Model file for the job. Use its own axes, mm. Face numbers are marked on the shaded views. A direction names the side the tool comes from. Give positions to 0.01 mm unless a question says otherwise; leave off trailing zeros. Order: outer loops, then holes, each group sorted by start corner. A loop starts at its lowest first (then second) coordinate and runs counter-clockwise, first axis right, second up. Notation, with made-up numbers: (78.5, 36) - (116.5, 36) arc R7 ccw to (116.5, 41) - close; hole circle Ø3 at (11.25, 52). An arc over 180 degrees is marked (long way). Use CSV: the item, a comma, the result in double quotes. Start each with the question number.
(1) Band-saw the part on A-A, the plane z = 8. Give the cut face in (x, y).
(2) Band-saw the part on C-C, the plane y = -35. Give the cut face in (x, z).
(3) Pull direction Z, two halves, no side cores. Call the marked faces 5, 6 and 7: +Z half, -Z half, draft (parallel to the pull), parting line (faces both ways), or undercut.
(4) Drop flat-ended pins along their axis: pin 1 Ø3 at (x, y) = (-18, -20) entering from +Z; pin 2 Ø1.2 at (x, y) = (18, -18) entering from -Z; pin 3 Ø7.5 at (y, z) = (-5, 19.5) entering from -X; pin 4 Ø0.9 at (y, z) = (-8.5, -12) entering from +X. Give the stop position or say it passes through.
(5) Tool access for the marked faces 1, 2, 3 and 4: list every direction of +Z, -Z, +X, -X, +Y, -Y with a clear straight run to the whole face (end or side of a thin tool).
(6) Probe L1, parallel to Z at x = 18.35, y = -35; L2, parallel to X at y = -10, z = -5; L3, parallel to Z at x = 4.5, y = -11. List the from-to ranges inside material, lowest first.
(7) Band-saw the part on D-D, the plane x = 11. Give the cut face in (y, z), then the cut area to 3 significant figures.
(8) Band-saw the part on B-B, the plane y = -10.5. Give the cut face in (x, z), then the cut area to 3 significant figures.
from build123d import *

# Parameters (mm, degrees)
SKETCH_1_W                       = 35
SKETCH_1_H                       = 22
SM_BASE_FLANGE_1_DEPTH           = 1
SM_EDGE_FLANGE_1_STRIP_W         = 5
SM_EDGE_FLANGE_1_STRIP_H         = 1
SM_EDGE_FLANGE_1_STRIP_CUT_DEPTH = 22
SM_EDGE_FLANGE_1_DEPTH           = 22
SM_EDGE_FLANGE_2_STRIP_W         = 5
SM_EDGE_FLANGE_2_STRIP_H         = 1
SM_EDGE_FLANGE_2_STRIP_CUT_DEPTH = 22
SM_EDGE_FLANGE_2_DEPTH           = 22
SM_EDGE_FLANGE_3_DEPTH           = 34
EXTRUDE_1_DEPTH                  = 22
SM_EDGE_FLANGE_4_DEPTH           = 20
SM_EDGE_FLANGE_5_STRIP_CUT_DEPTH = 22
SM_EDGE_FLANGE_5_DEPTH           = 22
CUT_EXTRUDE_1_DEPTH              = 22
SKETCH_27_R                      = 1.05
CUT_EXTRUDE_2_DEPTH              = 22


# Sheet-metal steps are written as plain solids
with BuildPart() as part:
    # Sketch 1 → 基体-法兰1 (new body)
    with BuildSketch(Plane(origin=(0, 0, 0), x_dir=(1, 0, 0), z_dir=(0, 1, 0))):
        Rectangle(SKETCH_1_W, SKETCH_1_H)
    extrude(amount=-SM_BASE_FLANGE_1_DEPTH)

    # 边线-法兰1 strip (across the edge) → 边线-法兰1 strip cut (cut)
    with BuildSketch(Plane(origin=(-17.5, -1, 11), x_dir=(1, 0, 0), z_dir=(0, 0, -1))):
        with Locations((-2, -0.5)):
            Rectangle(SM_EDGE_FLANGE_1_STRIP_W, SM_EDGE_FLANGE_1_STRIP_H)
    extrude(amount=SM_EDGE_FLANGE_1_STRIP_CUT_DEPTH, mode=Mode.SUBTRACT)

    # 边线-法兰1 section (across the edge) → 边线-法兰1 (add)
    with BuildSketch(Plane(origin=(-17.5, -1, 11), x_dir=(1, 0, 0), z_dir=(0, 0, -1))):
        with BuildLine():
            Line((-1, 0.5), (-1, 19))
            Line((-1, 19), (0, 19))
            Line((0, 19), (0, 0.5))
            ThreePointArc((0, 0.5), (0.146446609, 0.146446609), (0.5, 0))
            Line((0.5, 0), (0.5, -1))
            ThreePointArc((0.5, -1), (-0.560660172, -0.560660172), (-1, 0.5))
        make_face()
    extrude(amount=SM_EDGE_FLANGE_1_DEPTH)

    # 边线-法兰2 strip (across the edge) → 边线-法兰2 strip cut (cut)
    with BuildSketch(Plane(origin=(17.5, -1, -11), x_dir=(-1, 0, 0), z_dir=(0, 0, 1))):
        with Locations((-2, -0.5)):
            Rectangle(SM_EDGE_FLANGE_2_STRIP_W, SM_EDGE_FLANGE_2_STRIP_H)
    extrude(amount=SM_EDGE_FLANGE_2_STRIP_CUT_DEPTH, mode=Mode.SUBTRACT)

    # 边线-法兰2 section (across the edge) → 边线-法兰2 (add)
    with BuildSketch(Plane(origin=(17.5, -1, -11), x_dir=(-1, 0, 0), z_dir=(0, 0, 1))):
        with BuildLine():
            Line((-1, 0.5), (-1, 37))
            Line((-1, 37), (0, 37))
            Line((0, 37), (0, 0.5))
            ThreePointArc((0, 0.5), (0.146446609, 0.146446609), (0.5, 0))
            Line((0.5, 0), (0.5, -1))
            ThreePointArc((0.5, -1), (-0.560660172, -0.560660172), (-1, 0.5))
        make_face()
    extrude(amount=SM_EDGE_FLANGE_2_DEPTH)

    # 边线-法兰3 section (across the edge) → 边线-法兰3 (add)
    with BuildSketch(Plane(origin=(-17, -1, -11.7366), x_dir=(0, 0, 1), z_dir=(1, 0, 0))):
        with BuildLine():
            Line((-1, 0.7366), (-1, 14.7366))
            Line((-1, 14.7366), (0, 14.7366))
            Line((0, 14.7366), (0, 0.7366))
            ThreePointArc((0, 0.7366), (0.215745145, 0.215745145), (0.7366, 0))
            Line((0.7366, 0), (0.7366, -1))
            ThreePointArc((0.7366, -1), (-0.491361636, -0.491361636), (-1, 0.7366))
        make_face()
    extrude(amount=SM_EDGE_FLANGE_3_DEPTH)

    # 草图19 → 凸台-拉伸1 (add)
    with BuildSketch(Plane.XY.offset(11)):
        Polygon((0, 0), (10, 0), (10, -1), (-10, -1), (-10, 0), align=None)
    extrude(amount=EXTRUDE_1_DEPTH)

    # 边线-法兰4 section (across the edge) → 边线-法兰4 (add)
    with BuildSketch(Plane(origin=(10, -1, 33.7366), x_dir=(0, 0, -1), z_dir=(-1, 0, 0))):
        with BuildLine():
            Line((-1, 0.7366), (-1, 14))
            Line((-1, 14), (0, 14))
            Line((0, 14), (0, 0.7366))
            ThreePointArc((0, 0.7366), (0.215745145, 0.215745145), (0.7366, 0))
            Line((0.7366, 0), (0.7366, -1))
            ThreePointArc((0.7366, -1), (-0.491361636, -0.491361636), (-1, 0.7366))
        make_face()
    extrude(amount=SM_EDGE_FLANGE_4_DEPTH)

    # 边线-法兰5 strip (across the edge) → 边线-法兰5 strip cut (cut)
    with BuildSketch(Plane(origin=(-18.5, -20, -11), x_dir=(-0.8660254037844398, 0.4999999999999981, 0), z_dir=(0, 0, 1))):
        Polygon((-3.503939716, 4.069001615), (-0.767339716, -0.670928625), (0.098685688, -0.170928625), (-2.637914312, 4.569001615), align=None)
    extrude(amount=SM_EDGE_FLANGE_5_STRIP_CUT_DEPTH, mode=Mode.SUBTRACT)

    # 边线-法兰5 section (across the edge) → 边线-法兰5 (add)
    with BuildSketch(Plane(origin=(-18.5, -20, -11), x_dir=(-0.8660254037844398, 0.4999999999999981, 0), z_dir=(0, 0, 1))):
        with BuildLine():
            Line((-1, 0.197371375), (-1, 8.732050808))
            Line((-1, 8.732050808), (0, 8.732050808))
            Line((0, 8.732050808), (0, 0.197371375))
            ThreePointArc((0, 0.197371375), (0.025099036, 0.006725267), (0.098685688, -0.170928625))
            Line((0.098685688, -0.170928625), (-0.767339716, -0.670928625))
            ThreePointArc((-0.767339716, -0.670928625), (-0.94082679, -0.252093779), (-1, 0.197371375))
        make_face()
    extrude(amount=SM_EDGE_FLANGE_5_DEPTH)

    # 草图26 → 切除-拉伸1 (cut)
    with BuildSketch(Plane(origin=(-5.214745962, 3.010734985, 0), x_dir=(0, 0, 1), z_dir=(-0.8660254037844398, 0.49999999999999806, 0))):
        with BuildLine():
            Line((-4.3, -29.902558883), (4.3, -29.902558883))
            ThreePointArc((4.3, -29.902558883), (5.5, -31.102558883), (4.3, -32.302558883))
            Line((4.3, -32.302558883), (-4.3, -32.302558883))
            ThreePointArc((-4.3, -32.302558883), (-5.5, -31.102558883), (-4.3, -29.902558883))
        make_face()
    extrude(amount=-CUT_EXTRUDE_1_DEPTH, mode=Mode.SUBTRACT)

    # 草图27 → 切除-拉伸2 (cut)
    with BuildSketch(Plane(origin=(18.5, 0, 0), x_dir=(0, 0, -1), z_dir=(1, 0, 0))):
        with Locations(Location((8, -35, 0), (0, 0, 90))):
            Circle(SKETCH_27_R)
        with Locations(Location((-8, -35, 0), (0, 0, 90))):
            Circle(SKETCH_27_R)
    extrude(amount=-CUT_EXTRUDE_2_DEPTH, mode=Mode.SUBTRACT)


solid = part.part
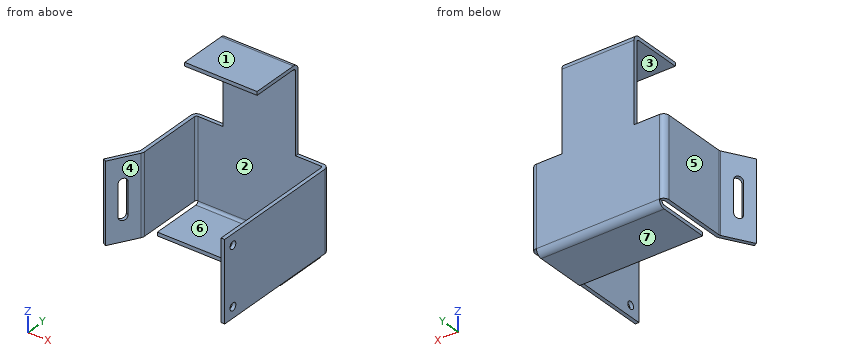
Answer block:
1,outline,"(-22.87, -27.56) - (-22, -28.06) - (-17.73, -20.67) arc R1.74 ccw to (-17.5, -19.8) - (-17.5, -1.5) arc R0.5 cw to (-17, -1) - (17, -1) arc R0.5 cw to (17.5, -1.5) - (17.5, -33.95) - (18.5, -33.95) - (18.5, -1.5) arc R1.5 ccw to (17, 0) - (-17, 0) arc R1.5 ccw to (-18.5, -1.5) - (-18.5, -19.8) arc R0.74 cw to (-18.6, -20.17) - close; (17.5, -38) - (18.5, -38) - (18.5, -36.05) - (17.5, -36.05) - close"
2,outline,"(17.5, -11) - (18.5, -11) - (18.5, -9.05) - (17.5, -9.05) - close; (17.5, -6.95) - (18.5, -6.95) - (18.5, 6.95) - (17.5, 6.95) - close; (17.5, 9.05) - (18.5, 9.05) - (18.5, 11) - (17.5, 11) - close"
3,face 5,"draft"
3,face 6,"undercut"
3,face 7,"-Z half"
4,pin 1,"stops at z = 11"
4,pin 2,"stops at z = -11"
4,pin 3,"passes through"
4,pin 4,"stops at x = 17"
5,face 1,"+Z, +X, -X, +Y, -Y"
5,face 2,"-Y"
5,face 3,"+X, -X, -Y"
5,face 4,"+Z, -Z, -Y"
6,L1,"z = -11 to -9.05, -6.95 to 6.95, 9.05 to 11"
6,L2,"x = -18.5 to -17.5, 17.5 to 18.5"
6,L3,"z = -12.74 to -11.74, 33.74 to 34.74"
7,outline,"(-15.74, -12.74) - (-1.74, -12.74) arc R1.74 ccw to (0, -11) - (0, 11) - (-1, 11) - (-1, -11) arc R0.74 cw to (-1.74, -11.74) - (-15.74, -11.74) - close"
7,area,"37.9 mm2"
8,outline,"(-18.5, -11) - (-17.5, -11) - (-17.5, 11) - (-18.5, 11) - close; (-17, -12.74) - (17, -12.74) - (17, -11.74) - (-17, -11.74) - close; (-10, 33.74) - (10, 33.74) - (10, 34.74) - (-10, 34.74) - close; (17.5, -11) - (18.5, -11) - (18.5, 11) - (17.5, 11) - close"
8,area,"98.0 mm2"
